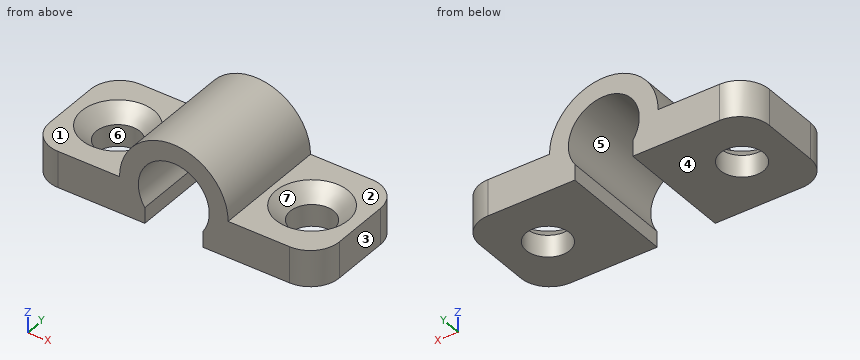
```python
from build123d import *

# Parameters (mm, degrees)
PAD_DEPTH    = 8
SKETCH001_R  = 1.5
POCKET_DEPTH = 2.501
CHAMFER_SIZE = 1
FILLET_R     = 2


with BuildPart() as part:
    # Sketch → Pad (new body)
    with BuildSketch(Plane.XZ):
        with BuildLine():
            ThreePointArc((12, 1.084903), (10, 4.95), (8, 1.084903))
            Line((8, 1.084903), (8, 0))
            Line((0, 0), (8, 0))
            Line((0, 2.5), (0, 0))
            Line((6.25, 2.5), (0, 2.5))
            ThreePointArc((13.75, 2.5), (10, 6.25), (6.25, 2.5))
            Line((20, 2.5), (13.75, 2.5))
            Line((20, 0), (20, 2.5))
            Line((12, 0), (20, 0))
            Line((12, 1.084903), (12, 0))
        make_face()
    extrude(amount=PAD_DEPTH)

    # Sketch001 → Pocket (cut, through all)
    with BuildSketch(Plane.XY.offset(2.5)):
        with Locations((3.3, -4)):
            Circle(SKETCH001_R)
        with Locations((16.7, -4)):
            Circle(SKETCH001_R)
    extrude(amount=-POCKET_DEPTH, mode=Mode.SUBTRACT)

    # Chamfer
    chamfer_edges = [part.edges().sort_by_distance(p)[0] for p in [
        (1.8, -4, 2.5),
        (15.2, -4, 2.5),
    ]]
    chamfer(chamfer_edges, length=CHAMFER_SIZE)

    # Fillet
    fillet_edges = [part.edges().sort_by_distance(p)[0] for p in [
        (0, -8, 1.25),
        (20, -8, 1.25),
        (20, 0, 1.25),
        (0, 0, 1.25),
    ]]
    fillet(fillet_edges, radius=FILLET_R)


solid = part.part
```
Input: part model. Units: mm. Frame: model coordinates. Face numbers are marked on the shaded views. A direction names the side the tool comes from. Coordinates: 2 decimals unless noted, no trailing zeros. Order: outer loops, then holes, each group sorted by start corner. A loop starts at its lowest first (then second) coordinate and runs counter-clockwise, first axis right, second up. Notation, with made-up numbers: (72, 57.25) - (105, 57.25) arc R18 cw to (105, 70.25) - close; hole circle Ø11 at (36, 43.25). An arc over 180 degrees is marked (long way). Return JSON: item names as keys, results as strings.
Q1. Ray query, probe 1 along X at (y, z) = (-7, 2.75); probe 2 along X at (y, z) = (-5, 4); probe 3 along Z at (x, y) = (12.25, -5.5). Return the intervals inside material, ascending.
The answers:
{"probe 1": "x = 6.26 to 7.56, 12.44 to 13.74", "probe 2": "x = 6.56 to 8.06, 11.94 to 13.44", "probe 3": "z = 0 to 1.53, 3.47 to 5.5"}
Q2. Cut plane C-C (z = 4.5). Return loops of the section in (x, y), then the cut area to 3 significant figures.
The answers:
{"outline": "(6.83, -8) - (8.58, -8) - (8.58, 0) - (6.83, 0) - close; (11.42, -8) - (13.17, -8) - (13.17, 0) - (11.42, 0) - close", "area": "28.1 mm2"}
Q3. Cut plane D-D (y = -5). State how many separate pieces and enclosed holes the cut face has, then the cut area to 3 significant figures.
The answers:
{"separate pieces": "3", "enclosed holes": "0", "area": "38.2 mm2"}
Q4. Cut plane B-B (x = 16.7). Return loops of the section in (y, z), then the cut area to 3 significant figures.
The answers:
{"outline": "(-8, 0) - (-5.5, 0) - (-5.5, 1.5) - (-6.5, 2.5) - (-8, 2.5) - close; (-2.5, 0) - (0, 0) - (0, 2.5) - (-1.5, 2.5) - (-2.5, 1.5) - close", "area": "11.5 mm2"}
Q5. First-contact query: pin 1 (3 mm diameter, centred on x = 4, y = -4, fed in from +Z); pin 2 (1.5 mm diameter, centred on y = -3, z = 5.5, fed in from +X); pin 3 (4 mm diameter, centred on x = 3.3, y = -4, fed in from +Z). Flat tips, straight axial feed; report the tip coordinate or a pass-through.
The answers:
{"pin 1": "stops at z = 2.2", "pin 2": "stops at x = 13", "pin 3": "stops at z = 2"}
Q6. Draft query along Z for the marked faces 4, 5, 6 and 7. Return one class per face: +Z half, -Z half, draft (parallel to the pull), parting line (faces both ways), or undercut.
The answers:
{"face 4": "-Z half", "face 5": "undercut", "face 6": "draft", "face 7": "+Z half"}
Q7. Cut plane A-A (z = 0.5). Return loops of the section in (x, y).
The answers:
{"outline": "(0, -6) arc R2 ccw to (2, -8) - (8, -8) - (8, 0) - (2, 0) arc R2 ccw to (0, -2) - close; (12, -8) - (18, -8) arc R2 ccw to (20, -6) - (20, -2) arc R2 ccw to (18, 0) - (12, 0) - close; hole circle Ø3 at (3.3, -4); hole circle Ø3 at (16.7, -4)"}
Q8. Access query for the marked faces 1, 2 and 3. Directions: +Z, -Z, +X, -X, +Y, -Y. A direction counts if a zero-diameter tool reaches every point of the face in a straight line with its end or side. Return the directions, or none.
The answers:
{"face 1": "+Z, -X, +Y, -Y", "face 2": "+Z, +X, +Y, -Y", "face 3": "+Z, -Z, +X, +Y, -Y"}
